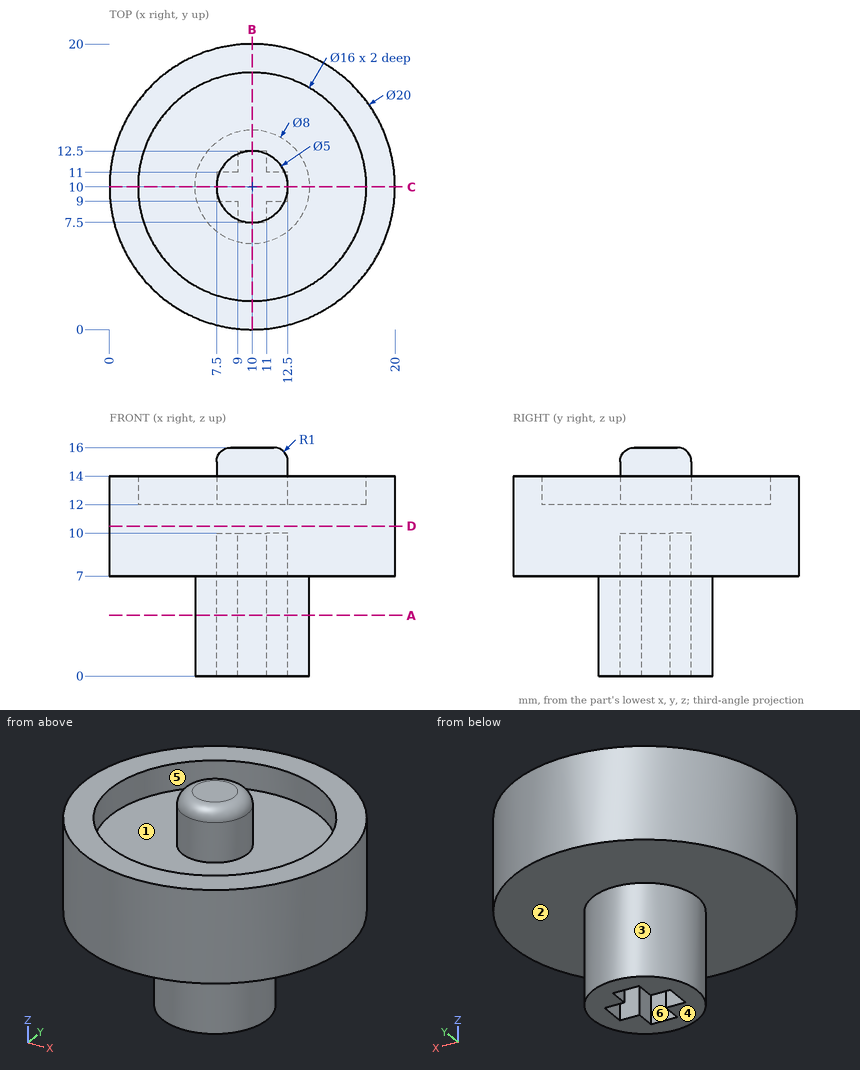
Print and shaded views of the part. All mm, measured from the part's lowest x, y and z. A direction names the side the tool comes from. Coordinates: 2 decimals unless noted, no trailing zeros. Write each loop counter-clockwise with the first axis right and the second up, starting at its lowest first coordinate (ties: lowest second). Pieces come first, ordered by that corner, then holes.
(1) Flat gauge pins, fed straight in: pin 1 (1.5 mm diameter, centred on x = 10.5, z = 3.5, fed in from +Y); pin 2 (1.6 mm diameter, centred on x = 12, z = 6, fed in from -Y); pin 3 (12 mm diameter, centred on x = 3, y = 17.5, fed in from -Z). Where does each tip first touch, or does it go through?
(2) 3-axis set-ups, long thin cutter, end or side, ignore diameter. For the marked faces 4, 5 and 6: which of +Z, -Z, +X, -X, +Y, -Y reach the whole face in a straight line?
(3) Drill centre lines: probe 1 along Y at (x, z) = (10, 13.5); probe 2 along Z at (x, y) = (11.75, 16.75); probe 3 along Z at (x, y) = (5, 3.5). Where is each one in solid material? Low to high.
(4) Two-plate mould, pull along Y, no slides. Class the marked faces 1, 2 and 3: +Y half, -Y half, draft (parallel to the pull), parting line (faces both ways), or undercut.
(5) Cut at B-B, the plane x = 10. List the corners of the cut face in (y, z).
(6) Cut at D-D, the plane z = 10.5. List the corners of the cut face in (x, y).
(7) Cut at A-A, the plane z = 4.25. List the corners of the cut face in (x, y).
Geometry says:
1. pin 1: stops at y = 14
1. pin 2: stops at y = 6.18
1. pin 3: stops at z = 7
2. face 4: -Z, +X, -X, +Y, -Y
2. face 5: +Z
2. face 6: -Z
3. probe 1: y = 0 to 2, 7.5 to 12.5, 18 to 20
3. probe 2: z = 7 to 12
3. probe 3: z = 7 to 14
4. face 1: undercut
4. face 2: draft
4. face 3: parting line
5. outline: (0, 7) - (6, 7) - (6, 0) - (7.5, 0) - (7.5, 10) - (12.5, 10) - (12.5, 0) - (14, 0) - (14, 7) - (20, 7) - (20, 14) - (18, 14) - (18, 12) - (12.5, 12) - (12.5, 15) arc R1 ccw to (11.5, 16) - (8.5, 16) arc R1 ccw to (7.5, 15) - (7.5, 12) - (2, 12) - (2, 14) - (0, 14) - close
6. outline: circle Ø20 at (10, 10)
7. outline: circle Ø8 at (10, 10); hole (7.5, 9) - (9, 9) - (9, 7.5) - (11, 7.5) - (11, 9) - (12.5, 9) - (12.5, 11) - (11, 11) - (11, 12.5) - (9, 12.5) - (9, 11) - (7.5, 11) - close
